Verification items for the finished model (mm, model axes). A direction names the side the tool comes from. Round coordinates to 2 decimals unless told otherwise and drop trailing zeros. Write each loop counter-clockwise with the first axis right and the second up, starting at its lowest first coordinate (ties: lowest second). Pieces come first, ordered by that corner, then holes. Notation, with made-up numbers: (-8.5, 10.25) - (35.5, 10.25) arc R18 cw to (35.5, 26.25) - close; hole circle Ø9 at (52, 74.25). An arc over 180 degrees is marked (long way). Answer as a JSON object with one key per item and string values.
```python
from build123d import *

# Parameters (mm, degrees)
F0_W     = 40
F0_H     = 20
F1_DEPTH = 25


with BuildPart() as f1:
    # F0 (on Top) → F1 (new body)
    with BuildSketch(Plane.XY):
        with Locations((-74.290519, 33.515131)):
            Rectangle(F0_W, F0_H)
    extrude(amount=F1_DEPTH)

    # F2 (on face) → F3 (revolve)
    with BuildSketch(Plane.XY.offset(25)):
        Polygon((-71.290519, 37.890665), (-74.290519, 39.622715), (-77.290519, 37.890665), (-77.290519, 34.426563), (-74.290519, 32.694512), (-71.290519, 34.426563), align=None)
    revolve(axis=Axis((-74.290519, 23.515131, 25), (1, 0, 0)))


solid = f1.part
```
Q1. Material ranges on line 1 along Y through (x, z) = (-63.5, 6.5); line 2 along X through (y, z) = (36, 29.5); line 3 along Z through (x, y) = (-66.5, 33), recorded low to high. Write a range as [from, to].
Geometry check:
{"line 1": "y = [23.52, 43.52]", "line 2": "x = [-77.29, -71.29]", "line 3": "z = [0, 25]"}
Q2. Section check B-B, the plane x = -89.5. Record the cut outline in (y, z), then the cut area to 3 significant figures.
Geometry check:
{"outline": "(23.52, 0) - (43.52, 0) - (43.52, 25) - (23.52, 25) - close", "area": "500 mm2"}
Q3. Set-up check for faces 1 (the conical face through (-71.478, 13.617, 35.574)), 2 (the flat face through (-71.291, 18, 35)): record each of +Z, -Z, +X, -X, +Y, -Y from which the full face is reachable in a straight line by a thin tool's end or side.
Geometry check:
{"face 1": "+X", "face 2": "+Z, +X, -Y"}
Q4. Gauge pin test, flat ends, axial feed: P1, Ø12, axis at x = -81.5, y = 34, coming from the +Z side; P2, Ø5, axis at x = -58.5, z = 11, coming from the -Y side; P3, Ø16, axis at x = -73, y = 32.5, coming from the +Z side; P4, Ø6, axis at y = 23, z = 22.5, coming from the +X side. Record the tip position at first contact, or that the pin passes through.
Geometry check:
{"P1": "stops at z = 38.01", "P2": "stops at y = 23.52", "P3": "stops at z = 41.07", "P4": "stops at x = -54.29"}
Q5. Section check A-A, the plane z = 6.5. Record the cut outline in (x, y), then the cut area to 3 significant figures.
Geometry check:
{"outline": "(-94.29, 23.52) - (-54.29, 23.52) - (-54.29, 43.52) - (-94.29, 43.52) - close", "area": "800 mm2"}
Q6. Release check for a two-part mould opening along Z. For faces 3 (the conical face through (-74.103, 17.168, 31.78)), 4 (the flat face through (-75, 34, 0)), 5 (the flat face through (-77.291, 18, 35)) record: released by +Z, released by -Z, zero draft, split by the parting line, or undercut.
Geometry check:
{"face 3": "undercut", "face 4": "released by -Z", "face 5": "zero draft"}
